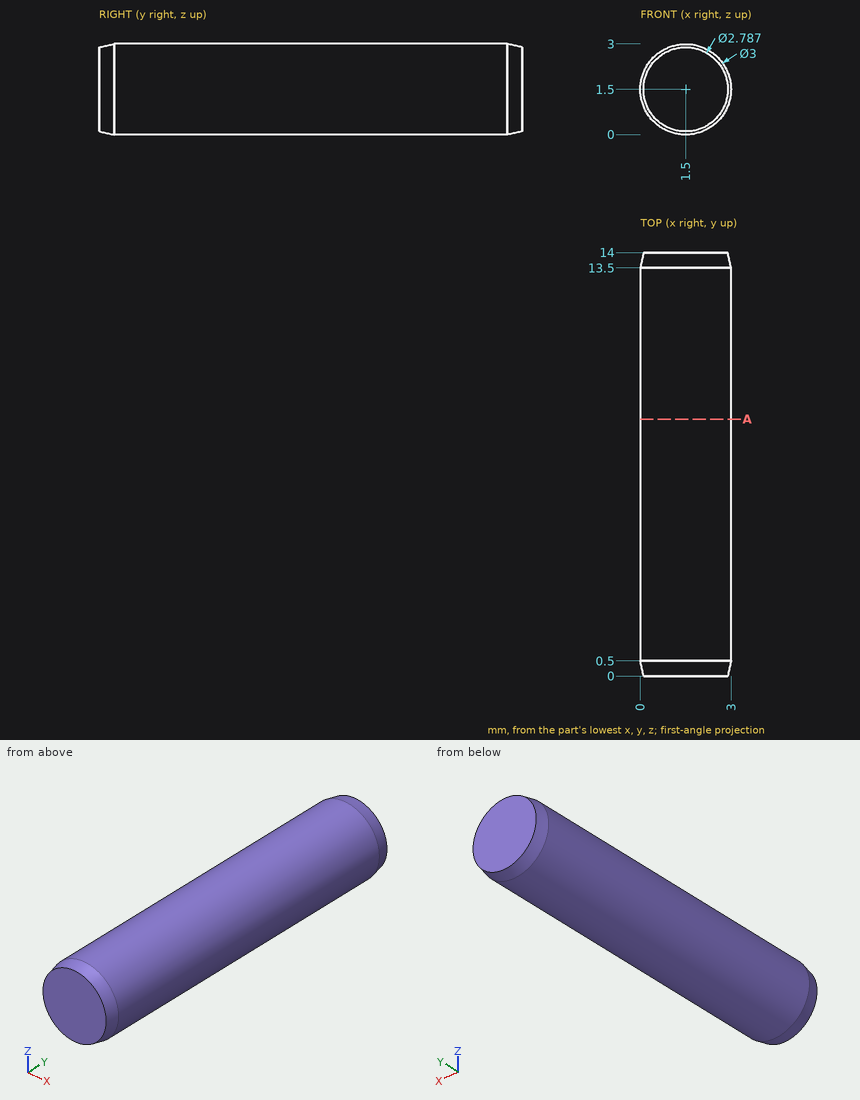
The figure shows three views and two pictorial views of one solid part (mm, origin at its lowest corner). Answer the questions. Coordinates: 2 decimals unless noted, no trailing zeros. Write each loop counter-clockwise with the first axis right and the second up, starting at its lowest first coordinate (ties: lowest second). Pieces come first, ordered by that corner, then holes. Notation, with made-up numbers: M 30,60 L 61,60 A22 cw 61,96 Z; hole C -37,44.5 d5. An arc over 180 degrees is marked long. Answer as CSV lines item,"result". Start each with the question number.
Item 1: Section A-A on y = 8.5 is taken. Write down the section's boundary in (x, z).
Item 2: Consider L1, parallel to X at y = 3.5, z = 1.4; L2, parallel to Z at x = 0.5, y = 2.25; L3, parallel to X at y = 9.5, z = 2.25. Determine where each line is inside the solid, lowest interval first.
Item 3: A flat-ended cylindrical pin translates along its axis: P1, Ø1, axis at x = 1.5, z = 1.5, coming from the -Y side. Find the tip coordinate at first contact, or state that the pin passes through.
Checks:
1,outline,"C 1.5,1.5 d3"
2,L1,"x = 0 to 3"
2,L2,"z = 0.38 to 2.62"
2,L3,"x = 0.2 to 2.8"
3,P1,"stops at y = 0"
